Design review of the part shown in the three views and the two pictorial views. Dimensions are in mm from the part's minimum x, y and z. A direction names the side the tool comes from. Coordinates: 2 decimals unless noted, no trailing zeros. Order: outer loops, then holes, each group sorted by start corner. A loop starts at its lowest first (then second) coordinate and runs counter-clockwise, first axis right, second up. Notation, with made-up numbers: M 60.5,-25.5 L 118.5,-25.5 A19 cw 118.5,-8.5 Z; hole C 87,79.25 d3. An arc over 180 degrees is marked long. Use CSV: the item, a comma, the result in double quotes.
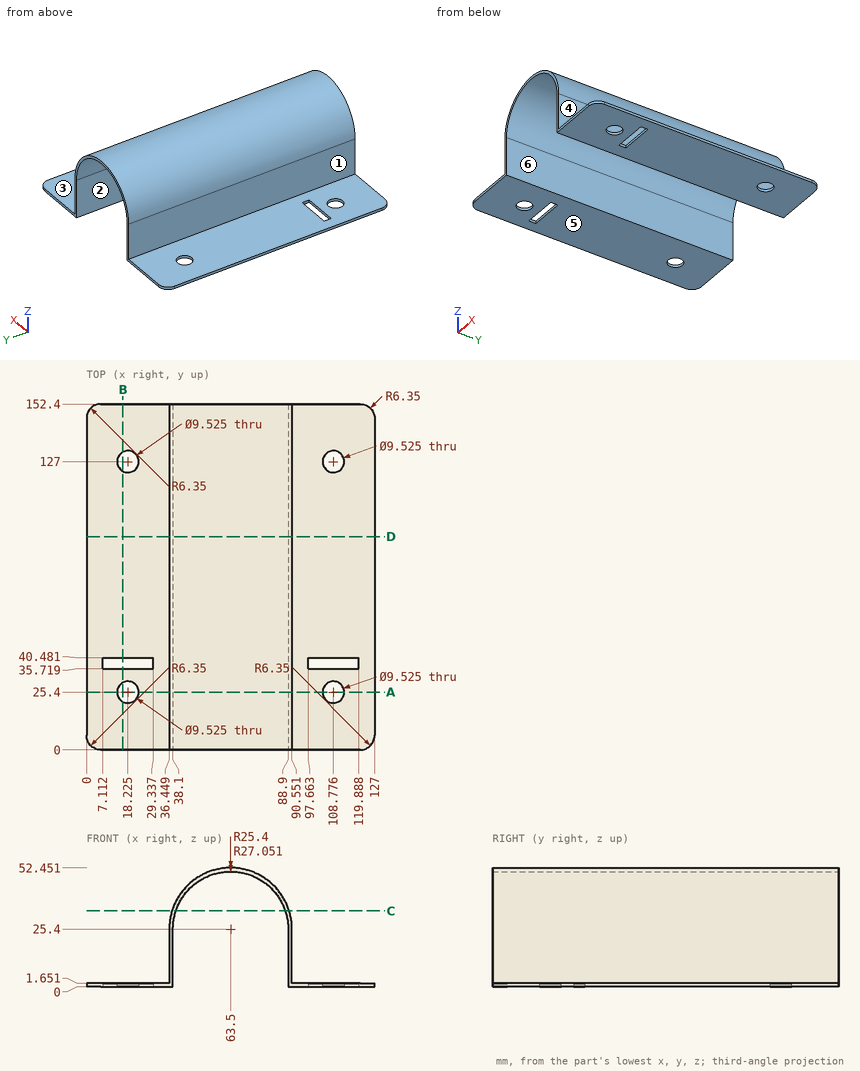
(1) The part is to be moulded in two halves that separate along X. For the marked faces 4, 5 and 6, say which applies: pulls with the +X half, pulls with the -X half, needs draft (parallel to the pull), parting line crosses it, or undercut.
The answers:
face 4,"pulls with the +X half"
face 5,"needs draft"
face 6,"undercut"
(2) Add section D-D on y = 94. State the section outline as (x, z) points.
The answers:
outline,"M 0,0 L 38.1,0 L 38.1,25.4 A25.4 cw 88.9,25.4 L 88.9,0 L 127,0 L 127,1.65 L 90.55,1.65 L 90.55,25.4 A27.05 ccw 36.45,25.4 L 36.45,1.65 L 0,1.65 Z"
(3) For the marked faces 1, 2 and 3, list the 3-axis set-ups (+Z, -Z, +X, -X, +Y, -Y) from which the entire face can be reached by the end or side of a thin tool; tool diameter is ignored.
The answers:
face 1,"+Z, -X, +Y, -Y"
face 2,"-Z, +Y, -Y"
face 3,"+Z, +X, +Y, -Y"
(4) Add section A-A on y = 25.4. State the section outline as (x, z) points.
The answers:
outline,"M 0,0 L 13.46,0 L 13.46,1.65 L 0,1.65 Z; M 22.99,0 L 38.1,0 L 38.1,25.4 A25.4 cw 88.9,25.4 L 88.9,0 L 104.01,0 L 104.01,1.65 L 90.55,1.65 L 90.55,25.4 A27.05 ccw 36.45,25.4 L 36.45,1.65 L 22.99,1.65 Z; M 113.54,0 L 127,0 L 127,1.65 L 113.54,1.65 Z"
(5) Add section B-B on x = 16. State the section outline as (y, z) points.
The answers:
outline,"M 0,0 L 21.19,0 L 21.19,1.65 L 0,1.65 Z; M 29.61,0 L 35.72,0 L 35.72,1.65 L 29.61,1.65 Z; M 40.48,0 L 122.79,0 L 122.79,1.65 L 40.48,1.65 Z; M 131.21,0 L 152.4,0 L 152.4,1.65 L 131.21,1.65 Z"
(6) Wall thickness on probe 1 along X at (y, z) = (18, 20.5); probe 2 along Z at (x, y) = (94.5, 118.5); probe 3 along X at (y, z) = (25, 26) (1 decimal): over which ranges is each line inside the solid? List them lowest first.
The answers:
probe 1,"x = 36.45 to 38.1, 88.9 to 90.55"
probe 2,"z = 0 to 1.65"
probe 3,"x = 36.5 to 38.1, 88.9 to 90.5"
(7) Add section C-C on z = 33.5. State the section outline as (x, y) points.
The answers:
outline,"M 37.69,0 L 39.43,0 L 39.43,152.4 L 37.69,152.4 Z; M 87.57,0 L 89.31,0 L 89.31,152.4 L 87.57,152.4 Z"
(8) Clearance check with flat-ended pins moving along their axes: P1, Ø4, axis at x = 62, y = 24.5, coming from the -Z side; P2, Ø8, axis at y = 135.5, z = 26, coming from the +X side; P3, Ø1, axis at x = 46.5, z = 41.5, coming from the +Y side; P4, Ø1, axis at x = 93, y = 103, coming from the +Z side. State where each tip first meets the part, or that it passes through.
The answers:
P1,"stops at z = 50.56"
P2,"stops at x = 90.55"
P3,"passes through"
P4,"stops at z = 1.65"
